Part model, mm, in its own coordinate system. Face numbers are marked on the shaded views. A direction names the side the tool comes from. Round coordinates to 2 decimals unless told otherwise and drop trailing zeros. Write each loop counter-clockwise with the first axis right and the second up, starting at its lowest first coordinate (ties: lowest second). Pieces come first, ordered by that corner, then holes. Notation, with made-up numbers: M 17,41 L 45,41 A20 cw 45,58 Z; hole C -2.5,88 d2. An arc over 180 degrees is marked long. Use a Markdown table: item, result. Add a question column.
1) Slice it at A-A on z = 25. Write the cut outline in (x, y).
2) Drop flat-ended pins along their axis: P1, Ø5, axis at y = 18, z = 18.5, coming from the -X side; P2, Ø1, axis at y = 13.5, z = 12, coming from the -X side; P3, Ø1.5, axis at x = -19, z = 12, coming from the -Y side; P4, Ø6, axis at y = -4.5, z = 25, coming from the +X side. Give the stop position or say it passes through.
3) Wall check: probe 1 along Z at (x, y) = (-4.5, 20.5); probe 2 along Y at (x, z) = (0, 17); probe 3 along X at (y, z) = (3.5, 20.5). Give the ranges that are in metal, low to high.
4) Which spindle directions (+Z, -Z, +X, -X, +Y, -Y) get a long thin tool onto all of the face, cutting with end or side? Do the marked faces 1, 2, 3, 4 and 5. Say none if no direction does.
5) Slice it at B-B on x = -17.5. Write the cut outline in (y, z).
6) Slice it at D-D on x = 18.5. Write the cut outline in (y, z), plus the area to 3 significant figures.
7) Slice it at C-C on z = 3.5. Write the cut outline in (x, y), plus the area to 3 significant figures.
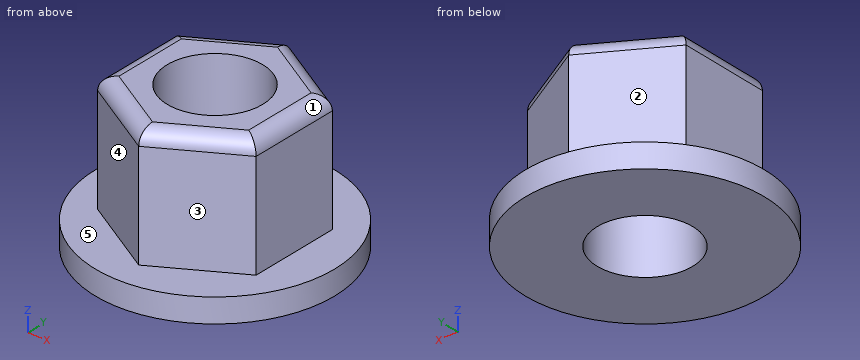
```python
from build123d import *

# Parameters (mm, degrees)
SKETCH2_R           = 25
BOSS_EXTRUDE1_DEPTH = 5
BOSS_EXTRUDE2_DEPTH = 25
FILLET6_R           = 3
SKETCH5_R           = 10
CUT_EXTRUDE1_DEPTH  = 31


with BuildPart() as part:
    # Sketch2 → Boss-Extrude1 (new body)
    with BuildSketch(Plane.XY):
        Circle(SKETCH2_R)
    extrude(amount=BOSS_EXTRUDE1_DEPTH)

    # Sketch3 → Boss-Extrude2 (add)
    with BuildSketch(Plane.XY.offset(5)):
        Polygon((16.644393052, -9.427942918), (16.487034598, 9.700495755), (-0.157358454, 19.128438672), (-16.644393052, 9.427942918), (-16.487034598, -9.700495755), (0.157358454, -19.128438672), align=None)
    extrude(amount=BOSS_EXTRUDE2_DEPTH)

    # Fillet6
    fillet6_edges = [part.edges().sort_by_distance(p)[0] for p in [
        (8.400875753, -14.278190795, 30),
        (16.565713825, 0.136276419, 30),
        (8.164838072, 14.414467214, 30),
        (-8.400875753, 14.278190795, 30),
        (-16.565713825, -0.136276419, 30),
        (-8.164838072, -14.414467214, 30),
    ]]
    fillet(fillet6_edges, radius=FILLET6_R)

    # Sketch5 → Cut-Extrude1 (cut, through all)
    with BuildSketch(Plane.XY.offset(30)):
        Circle(SKETCH5_R)
    extrude(amount=-CUT_EXTRUDE1_DEPTH, mode=Mode.SUBTRACT)


solid = part.part
```
Entries:
| question | item | result |
|---|---|---|
| 1 | outline | M -16.64,9.43 L -16.49,-9.7 L 0.16,-19.13 L 16.64,-9.43 L 16.49,9.7 L -0.16,19.13 Z; hole C 0,0 d20 |
| 2 | P1 | stops at x = -6.32 |
| 2 | P2 | stops at x = -10.57 |
| 2 | P3 | passes through |
| 2 | P4 | stops at x = 16.63 |
| 3 | probe 1 | z = 0 to 5 |
| 3 | probe 2 | y = -19.04 to -10, 10 to 19.04 |
| 3 | probe 3 | x = -16.6 to -9.37, 9.37 to 16.54 |
| 4 | face 1 | +Z, +X, +Y |
| 4 | face 2 | +Z, -X, +Y |
| 4 | face 3 | +Z, +X, -Y |
| 4 | face 4 | +Z, -X, -Y |
| 4 | face 5 | +Z |
| 5 | outline | M -17.85,0 L 17.85,0 L 17.85,5 L -17.85,5 Z |
| 6 | outline | M -16.82,0 L 16.82,0 L 16.82,5 L -16.82,5 Z |
| 6 | area | 168 mm^2 |
| 7 | outline | C 0,0 d50; hole C 0,0 d20 |
| 7 | area | 1,650 mm^2 |
